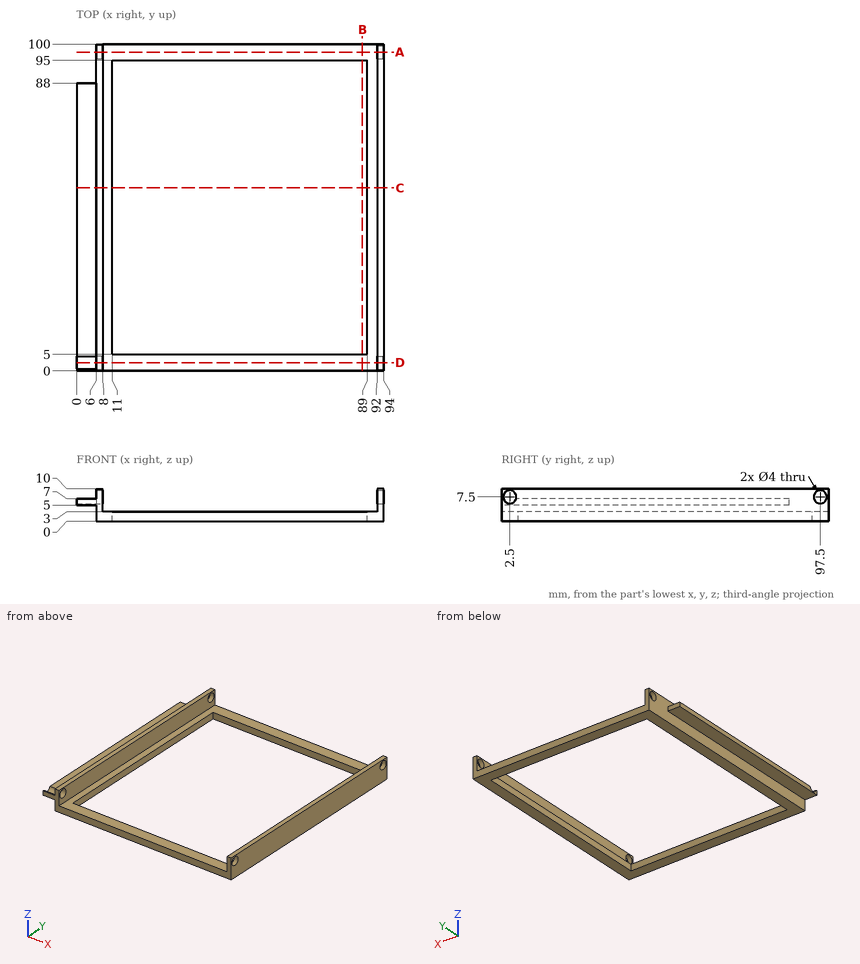
Can you work these out from the drawing? Everything is in mm from the part's minimum corner. Give positions to 0.01 mm unless a question says otherwise; leave off trailing zeros. Loops run counter-clockwise (first coordinate to the right, second up) from the corner with the lowest first, then second, coordinate; pieces in that order, holes last. Notation, with made-up numbers: (23.5, 71.5) - (82.5, 71.5) arc R14 ccw to (82.5, 98.5) - close; hole circle Ø2 at (83.5, 76.25). An arc over 180 degrees is marked (long way). Use one line per item in the form item = value.
1. I want a section at B-B (x = 87.5). Please give me the cut outline in (y, z).
Response values:
outline = (0, 0) - (5, 0) - (5, 3) - (0, 3) - close; (95, 0) - (100, 0) - (100, 3) - (95, 3) - close
2. I want a section at A-A (y = 97.5). Please give me the cut outline in (x, z), and give its area (3 significant figures).
Response values:
outline = (6, 0) - (94, 0) - (94, 5.5) - (92, 5.5) - (92, 3) - (8, 3) - (8, 5.5) - (6, 5.5) - close; (6, 9.5) - (8, 9.5) - (8, 10) - (6, 10) - close; (92, 9.5) - (94, 9.5) - (94, 10) - (92, 10) - close
area = 276 mm²
3. I want a section at C-C (y = 56). Please give me the cut outline in (x, z).
Response values:
outline = (0, 5) - (6, 5) - (6, 0) - (11, 0) - (11, 3) - (8, 3) - (8, 10) - (6, 10) - (6, 7) - (0, 7) - close; (89, 0) - (94, 0) - (94, 10) - (92, 10) - (92, 3) - (89, 3) - close
4. I need wall thicknesses on probe 1 along Z at (x, y) = (92.45, 97.5); probe 2 along Y at (x, z) = (21.5, 1.75); probe 3 along X at (y, z) = (28, 3.75). Which ranges of each line are inside material? Lowest first, please.
Response values:
probe_1 = 0 to 5.5, 9.5 to 10
probe_2 = 0 to 5, 95 to 100
probe_3 = 6 to 8, 92 to 94
5. I'm going to push flat-ended pins straight in: pin 1 Ø1 at (x, z) = (1.5, 5.5) entering from +Y; pin 2 Ø1 at (y, z) = (18, 2.5) entering from -X; pin 3 Ø6.5 at (x, y) = (1.5, 60.5) entering from -Z. Where does each tip first touch, or does it pass through?
Response values:
pin_1 = 88
pin_2 = 6
pin_3 = 5
6. I want a section at D-D (y = 2.5). Please give me the cut outline in (x, z).
Response values:
outline = (0, 5) - (6, 5) - (6, 0) - (94, 0) - (94, 5.5) - (92, 5.5) - (92, 3) - (8, 3) - (8, 5.5) - (0, 5.5) - close; (6, 9.5) - (8, 9.5) - (8, 10) - (6, 10) - close; (92, 9.5) - (94, 9.5) - (94, 10) - (92, 10) - close
